Could you check a few things on this drawing? It's one solid part, dimensions in mm from its lowest x, y, z. Give positions to 0.01 mm unless a question says otherwise; leave off trailing zeros. Loops run counter-clockwise (first coordinate to the right, second up) from the corner with the lowest first, then second, coordinate; pieces in that order, holes last. Notation, with made-up numbers: (-4, -38) - (50, -38) arc R20 ccw to (50, -9) - close; hole circle Ø10 at (-30, 20). An arc over 180 degrees is marked (long way). Put each result on its own line as item: value. Start each with the question number.
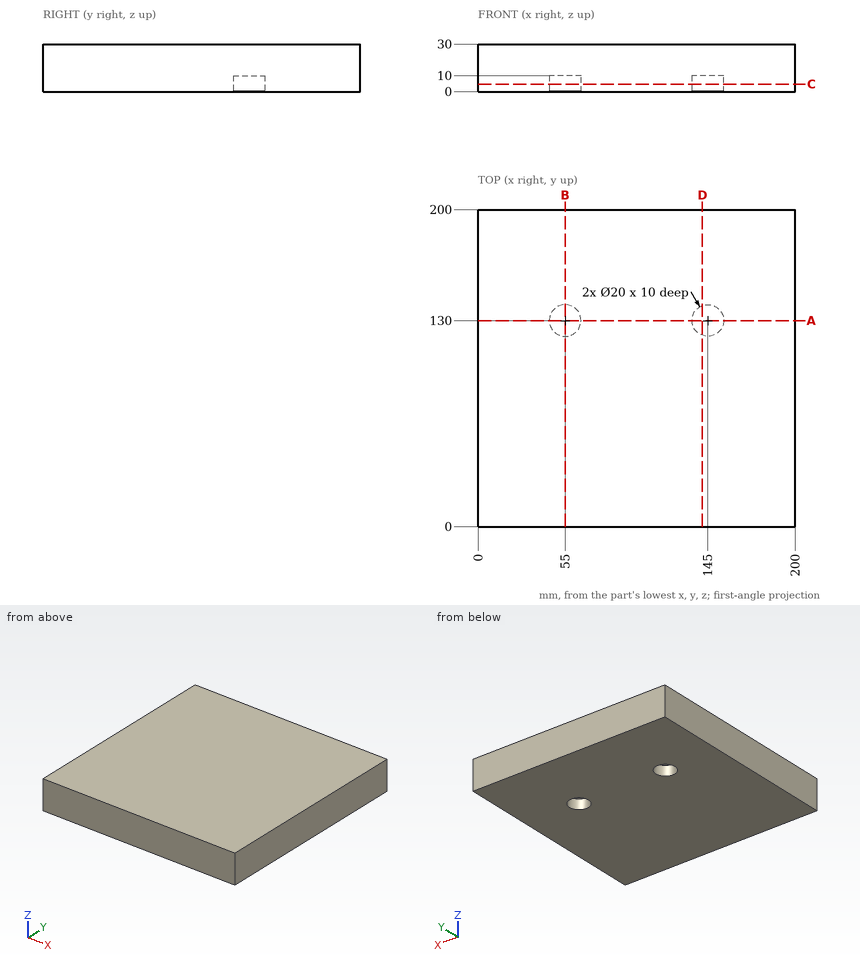
1) Suppose I cut it at B-B on x = 55. Please give me the cut outline in (y, z).
2) Suppose I cut it at D-D on x = 141.5. Please give me the cut outline in (y, z).
3) Suppose I cut it at A-A on y = 130. Please give me the cut outline in (x, z).
4) Suppose I cut it at C-C on z = 4.75. Please give me the cut outline in (x, y).
5) I need wall thicknesses on line 1 (Y direction, x = 145, z = 2). Which ranges of the line are inside material? Lowest first, please.
6) I'm going to push a flat-ended pin straight in: P1, Ø22, axis at x = 149.5, y = 128, coming from the -Z side. Where does the tip first touch, or does it pass through?
Ans:
1. outline: (0, 0) - (120, 0) - (120, 10) - (140, 10) - (140, 0) - (200, 0) - (200, 30) - (0, 30) - close
2. outline: (0, 0) - (120.63, 0) - (120.63, 10) - (139.37, 10) - (139.37, 0) - (200, 0) - (200, 30) - (0, 30) - close
3. outline: (0, 0) - (45, 0) - (45, 10) - (65, 10) - (65, 0) - (135, 0) - (135, 10) - (155, 10) - (155, 0) - (200, 0) - (200, 30) - (0, 30) - close
4. outline: (0, 0) - (200, 0) - (200, 200) - (0, 200) - close; hole circle Ø20 at (55, 130); hole circle Ø20 at (145, 130)
5. line 1: y = 0 to 120, 140 to 200
6. P1: stops at z = 0
